Work out the finished part from the listing and answer in its coordinate system (mm). Coordinates: 2 decimals unless noted, no trailing zeros. Order: outer loops, then holes, each group sorted by start corner. A loop starts at its lowest first (then second) coordinate and runs counter-clockwise, first axis right, second up.
1. Flat-ended cylindrical pins translate along their axes: pin 1 Ø1.6 at (y, z) = (-28.5, 1002) entering from +X; pin 2 Ø2 at (x, y) = (49.5, 17.5) entering from -Z; pin 3 Ø12 at (x, z) = (125.5, 1250.5) entering from +Y. Find the tip coordinate at first contact, or state that the pin passes through.
2. The part is cut by section A-A, the plane z = 313. Give the vertices of the cut face in (x, y), then the cut area to 3 significant figures.
3. Find the intervals of material crossed by probe 1 along X at (y, z) = (2, 770); probe 2 along Z at (x, y) = (93.5, -13.5); probe 3 along X at (y, z) = (-0.5, 407), in increasing order.
4. The part is cut by section B-B, the plane x = 58. Give the vertices of the cut face in (y, z), then the cut area to 3 significant figures.
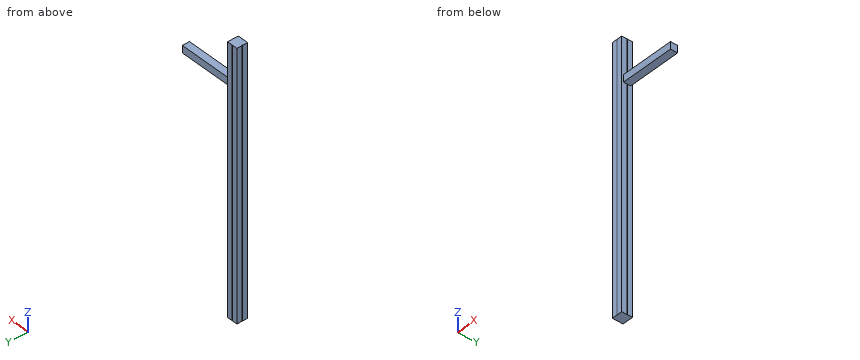
```python
from build123d import *

# Parameters (mm, degrees)
F0_W     = 60
F0_H     = 60
F1_DEPTH = 1465
F2_W     = 2
F2_H     = 2
F3_DEPTH = 1465
F4_W     = 40
F4_H     = 40
F5_DEPTH = 300


with BuildPart() as f1:
    # F0 (on Top) → F1 (new body)
    with BuildSketch(Plane.XY):
        Rectangle(F0_W, F0_H)
    extrude(amount=F1_DEPTH)

    # F2 (on face) → F3 (cut, through all)
    with BuildSketch(Plane.XY.offset(1465)):
        with Locations((0, 29)):
            Rectangle(F2_W, F2_H)
        with Locations((-29, 0)):
            Rectangle(F2_W, F2_H)
        with Locations((0, -29)):
            Rectangle(F2_W, F2_H)
        with Locations((29, 0)):
            Rectangle(F2_W, F2_H)
    extrude(amount=-F3_DEPTH, mode=Mode.SUBTRACT)

    # F4 (on face) → F5 (join)
    with BuildSketch(Plane.YZ.offset(30)):
        with Locations((0, 1245)):
            Rectangle(F4_W, F4_H)
    extrude(amount=F5_DEPTH)


solid = f1.part
```
Geometry says:
1. pin 1: stops at x = 30
1. pin 2: stops at z = 1225
1. pin 3: stops at y = 20
2. outline: (-30, -30) - (-1, -30) - (-1, -28) - (1, -28) - (1, -30) - (30, -30) - (30, -1) - (28, -1) - (28, 1) - (30, 1) - (30, 30) - (1, 30) - (1, 28) - (-1, 28) - (-1, 30) - (-30, 30) - (-30, 1) - (-28, 1) - (-28, -1) - (-30, -1) - close
2. area: 3,580 mm2
3. probe 1: x = -30 to 30
3. probe 2: z = 1225 to 1265
3. probe 3: x = -28 to 28
4. outline: (-20, 1225) - (20, 1225) - (20, 1265) - (-20, 1265) - close
4. area: 1,600 mm2
